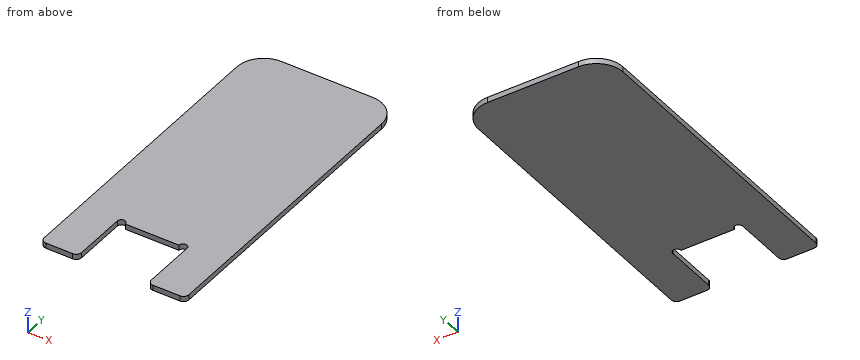
```python
from build123d import *

# Parameters (mm, degrees)
F1_DEPTH = 1


with BuildPart() as f1:
    # F0 (on Top) → F1 (new body)
    with BuildSketch(Plane.XY):
        with BuildLine():
            ThreePointArc((-13.5, 1), (-13.207107, 0.292893), (-12.5, 0))
            Line((-12.5, 0), (-7.5, 0))
            ThreePointArc((-7.5, 0), (-6.792893, 0.292893), (-6.5, 1))
            Line((-6.5, 1), (-6.5, 11))
            ThreePointArc((-6.5, 11), (-5.75, 11.75), (-5, 11))
            Line((-5, 11), (0, 11))
            Line((0, 11), (5, 11))
            ThreePointArc((5, 11), (5.75, 11.75), (6.5, 11))
            Line((6.5, 11), (6.5, 1))
            ThreePointArc((6.5, 1), (6.792893, 0.292893), (7.5, 0))
            Line((7.5, 0), (12.5, 0))
            ThreePointArc((12.5, 0), (13.207107, 0.292893), (13.5, 1))
            Line((13.5, 1), (13.5, 55))
            ThreePointArc((13.5, 55), (12.035534, 58.535534), (8.5, 60))
            Line((8.5, 60), (0, 60))
            Line((0, 60), (-8.5, 60))
            ThreePointArc((-8.5, 60), (-12.035534, 58.535534), (-13.5, 55))
            Line((-13.5, 55), (-13.5, 1))
        make_face()
    extrude(amount=F1_DEPTH)


solid = f1.part
```
Work out the finished part from the listing and answer in its coordinate system (mm). Give positions to 0.01 mm unless a question says otherwise; leave off trailing zeros. Loops run counter-clockwise (first coordinate to the right, second up) from the corner with the lowest first, then second, coordinate; pieces in that order, holes last. Notation, with made-up numbers: (-39.75, -20) -> (-15.75, -20) arc R22 ccw to (-15.75, 18) -> close; hole circle Ø2 at (70.25, 56.5). An arc over 180 degrees is marked (long way). Write item = value, one per line. Start each with the question number.
(1) Find section A-A on z = 0.85. Give the vertices of the cut face in (x, y), and give its area (3 significant figures).
(2) Find section C-C on x = 5.75. Give the vertices of the cut face in (y, z).
(3) Find section B-B on x = 0. Give the vertices of the cut face in (y, z).
(4) Find the intervals of material crossed by probe 1 along X at (y, z) = (3.5, 0.95); probe 2 along Y at (x, z) = (-1.5, 0.45); probe 3 along Y at (x, z) = (-5.75, 0.6), in increasing order. Write a range as from..to.
(5) Given pin 1 Ø0.5 at (x, z) = (0, 0.5) entering from -Y; pin 2 Ø10 at (x, y) = (-3.5, 51) entering from -Z, each flat-ended and moving along its own axis, determine where each tip first touches the part or whether it passes through.
From the geometry:
q1.outline = (-13.5, 1) arc R1 ccw to (-12.5, 0) -> (-7.5, 0) arc R1 ccw to (-6.5, 1) -> (-6.5, 11) arc R0.75 cw to (-5, 11) -> (5, 11) arc R0.75 cw to (6.5, 11) -> (6.5, 1) arc R1 ccw to (7.5, 0) -> (12.5, 0) arc R1 ccw to (13.5, 1) -> (13.5, 55) arc R5 ccw to (8.5, 60) -> (-8.5, 60) arc R5 ccw to (-13.5, 55) -> close
q1.area = 1,460 mm^2
q2.outline = (11.75, 0) -> (60, 0) -> (60, 1) -> (11.75, 1) -> close
q3.outline = (11, 0) -> (60, 0) -> (60, 1) -> (11, 1) -> close
q4.probe_1 = -13.5..-6.5, 6.5..13.5
q4.probe_2 = 11..60
q4.probe_3 = 11.75..60
q5.pin_1 = 11
q5.pin_2 = 0
